Check sheet for the modelled part. Datum: model origin and axes. Units: mm. Face numbers are marked on the shaded views. A direction names the side the tool comes from. Give positions to 0.01 mm unless a question says otherwise; leave off trailing zeros. Loops run counter-clockwise (first coordinate to the right, second up) from the corner with the lowest first, then second, coordinate; pieces in that order, holes last. Notation, with made-up numbers: (-33, 6.25) - (15, 6.25) arc R16 ccw to (15, 17.25) - close; hole circle Ø1 at (39.25, 19). An arc over 180 degrees is marked (long way). Answer in a Markdown table with one row per item. Add a question column.
(1) Sectioned sample at D-D on x = -8.5. Enter the section's corners in (y, z) (3 decimals), then the cut area to 3 significant figures.
(2) Sectioned sample at A-A on z = 0. Enter the section's corners in (x, y) (3 decimals).
(3) Set-up check for the marked faces 5, 6 and 7: record each of +Z, -Z, +X, -X, +Y, -Y from which the full face is reachable in a straight line by a thin tool's end or side.
(4) Draft check along Z on the marked faces 1, 2, 3 and 4. Enter one of: released by +Z, released by -Z, zero draft, split by the parting line, or undercut.
(5) Thickness scan on L1, parallel to Z at x = 1, y = -37; L2, parallel to Y at x = 1.5, z = 20 (3 decimals); L3, parallel to Y at x = -7.75, z = -22.5 (3 decimals). Record the ranges inside material, lowest first.
(6) Sectioned sample at C-C on z = -23. Enter the section's corners in (x, y) (3 decimals), then the cut area to 3 significant figures.
(7) Sectioned sample at B-B on y = 21.5. Enter the section's corners in (x, z).
(8) Go/stop test with flat-tipped pins: P1, Ø15, axis at y = -47.075, z = -25, coming from the +X side; P2, Ø25, axis at y = 14, z = -3.5, coming from the -X side; P3, Ø12, axis at x = -4, y = -1.5, coming from the +Z side; P4, Ø6, axis at x = -4, z = 16.5, coming from the -Y side. Record where each tip stops, or that it passes through.
from build123d import *

# Parameters (mm, degrees)
SKETCH1_W           = 50
SKETCH1_H           = 66.15
SKETCH1_R           = 11
SKETCH1_R_2         = 1.55
BOSS_EXTRUDE1_DEPTH = 4
SKETCH2_W           = 50
SKETCH2_H           = 4
BOSS_EXTRUDE2_DEPTH = 38
CHAMFER1_SIZE       = 10
CHAMFER1_SIZE2      = 4.663076582
BOSS_EXTRUDE3_START = -18
SKETCH3_R           = 5.25
SKETCH3_R_2         = 1.4
BOSS_EXTRUDE3_DEPTH = 24
SKETCH4_W           = 18
SKETCH4_H           = 50
CUT_EXTRUDE1_DEPTH  = 24
FILLET1_R           = 10
SKETCH5_W           = 25
SKETCH5_H           = 15
CUT_EXTRUDE2_DEPTH  = 86.707383725


with BuildPart() as part:
    # Sketch1 → Boss-Extrude1 (new body)
    with BuildSketch(Plane(origin=(0, 0, 0), x_dir=(0, 0, -1), z_dir=(1, 0, 0))):
        Rectangle(SKETCH1_W, SKETCH1_H)
        with Locations((0, 11.925)):
            Circle(SKETCH1_R, mode=Mode.SUBTRACT)
        with Locations((-15.5, 27.425)):
            Circle(SKETCH1_R_2, mode=Mode.SUBTRACT)
        with Locations((15.5, 27.425)):
            Circle(SKETCH1_R_2, mode=Mode.SUBTRACT)
        with Locations((15.5, -3.575)):
            Circle(SKETCH1_R_2, mode=Mode.SUBTRACT)
        with Locations((-15.5, -3.575)):
            Circle(SKETCH1_R_2, mode=Mode.SUBTRACT)
    extrude(amount=BOSS_EXTRUDE1_DEPTH)

    # Sketch2 → Boss-Extrude2 (add)
    with BuildSketch(Plane.ZY):
        with Locations((0, -31.075)):
            Rectangle(SKETCH2_W, SKETCH2_H)
    extrude(amount=BOSS_EXTRUDE2_DEPTH)

    # Chamfer1
    chamfer1_edges = [part.edges().sort_by_distance(p)[0] for p in [
        (0, -29.075, 0),
    ]]
    chamfer1_side = [part.faces().sort_by_distance(p)[0] for p in [
        (0, 0.490102601, 0),
    ]]
    chamfer(chamfer1_edges, length=CHAMFER1_SIZE, length2=CHAMFER1_SIZE2, reference=chamfer1_side[0])

    # Sketch3 → Boss-Extrude3 (add)
    with BuildSketch(Plane.ZY.offset(38).offset(BOSS_EXTRUDE3_START)):
        with BuildLine():
            Line((-25, -33.075), (-25, -38.075))
            ThreePointArc((-25, -38.075), (-32.372368399, -41.912812073), (-33.457233587, -50.15318129))
            Line((-33.457233587, -50.15318129), (-31.108002035, -49.298130932))
            ThreePointArc((-31.108002035, -49.298130932), (-18.994783039, -44.58755769), (-30.891000616, -49.822018701))
            Line((-30.891000616, -49.822018701), (-33.156770083, -50.878564356))
            ThreePointArc((-33.156770083, -50.878564356), (-29.835696475, -54.665523012), (-25, -56.075))
            Line((-25, -56.075), (-7.705679723, -56.075))
            ThreePointArc((-7.705679723, -56.075), (0, -74.925), (7.705679723, -56.075))
            Line((7.705679723, -56.075), (25, -56.075))
            ThreePointArc((25, -56.075), (29.835696475, -54.665523012), (33.156770083, -50.878564356))
            Line((33.156770083, -50.878564356), (30.891000616, -49.822018701))
            ThreePointArc((30.891000616, -49.822018701), (18.994783039, -44.58755769), (31.108002035, -49.298130932))
            Line((31.108002035, -49.298130932), (33.457233587, -50.15318129))
            ThreePointArc((33.457233587, -50.15318129), (32.372368399, -41.912812073), (25, -38.075))
            Line((25, -38.075), (25, -33.075))
            Line((25, -33.075), (-25, -33.075))
        make_face()
        with Locations((0, -63.925)):
            Circle(SKETCH3_R, mode=Mode.SUBTRACT)
        with Locations((0, -55.925)):
            Circle(SKETCH3_R_2, mode=Mode.SUBTRACT)
        with Locations((-8, -63.925)):
            Circle(SKETCH3_R_2, mode=Mode.SUBTRACT)
        with Locations((0, -71.925)):
            Circle(SKETCH3_R_2, mode=Mode.SUBTRACT)
        with Locations((8, -63.925)):
            Circle(SKETCH3_R_2, mode=Mode.SUBTRACT)
    extrude(amount=-BOSS_EXTRUDE3_DEPTH)

    # Sketch4 → Cut-Extrude1 (cut)
    with BuildSketch(Plane.XZ.offset(33.075)):
        with Locations((-29, 0)):
            Rectangle(SKETCH4_W, SKETCH4_H)
    extrude(amount=-CUT_EXTRUDE1_DEPTH, mode=Mode.SUBTRACT)

    # Fillet1
    fillet1_edges = [part.edges().sort_by_distance(p)[0] for p in [
        (-8, -56.075, -7.705679723),
        (-8, -56.075, 7.705679723),
    ]]
    fillet(fillet1_edges, radius=FILLET1_R)

    # Sketch5 → Cut-Extrude2 (cut, through all)
    with BuildSketch(Plane.ZY.offset(20)):
        with Locations((0, -41.575)):
            Rectangle(SKETCH5_W, SKETCH5_H)
    extrude(amount=-CUT_EXTRUDE2_DEPTH, mode=Mode.SUBTRACT)


solid = part.part
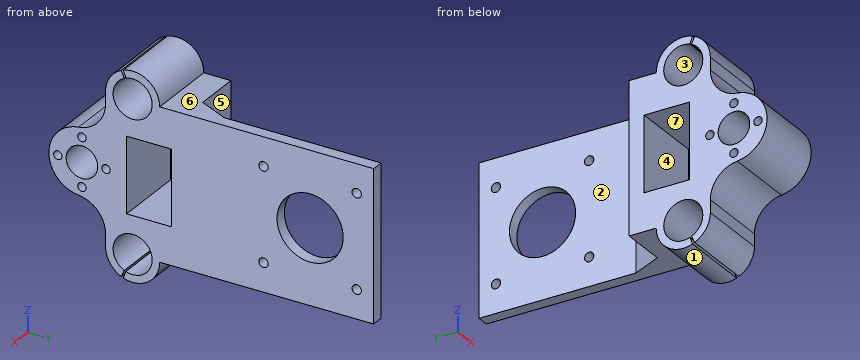
Reply:
| question | item | result |
|---|---|---|
| 1 | outline | (-65.051, -10.942) arc R10 cw to (-56.075, -20.89) - (-56.075, -25) arc R9 ccw to (-50.879, -33.157) - (-49.822, -30.891) arc R6.5 cw (long way) to (-49.298, -31.108) - (-50.153, -33.457) arc R9 ccw to (-38.075, -25) - (-29.075, -25) - (-29.075, 25) - (-38.075, 25) arc R9 ccw to (-50.153, 33.457) - (-49.298, 31.108) arc R6.5 cw (long way) to (-49.822, 30.891) - (-50.879, 33.157) arc R9 ccw to (-56.075, 25) - (-56.075, 20.89) arc R10 cw to (-65.051, 10.942) arc R11 ccw to start; hole circle Ø2.8 at (-71.925, 0); hole circle Ø10.5 at (-63.925, 0); hole circle Ø2.8 at (-63.925, -8); hole circle Ø2.8 at (-63.925, 8); hole circle Ø2.8 at (-55.925, 0); hole (-49.075, -12.5) - (-34.075, -12.5) - (-34.075, 12.5) - (-49.075, 12.5) - close |
| 1 | area | 1,250 mm^2 |
| 2 | outline | (-20, -74.925) - (4, -74.925) - (4, -73.325) - (-20, -73.325) - close; (-20, -70.525) - (4, -70.525) - (4, -69.175) - (-20, -69.175) - close; (-20, -58.675) - (4, -58.675) - (4, -57.325) - (-20, -57.325) - close; (-20, -54.525) - (4, -54.525) - (4, -49.075) - (-20, -49.075) - close; (-20, -34.075) - (4, -34.075) - (4, 0.925) - (0, 0.925) - (0, -19.075) - (-4.663, -29.075) - (-20, -29.075) - close; (0, 22.925) - (4, 22.925) - (4, 33.075) - (0, 33.075) - close |
| 3 | face 5 | +Z, -Z, -X, +Y |
| 3 | face 6 | +Z, +X, -X, +Y |
| 3 | face 7 | +X, -X |
| 4 | face 1 | released by -Z |
| 4 | face 2 | zero draft |
| 4 | face 3 | undercut |
| 4 | face 4 | undercut |
| 5 | L1 | -25 to -12.5, 12.5 to 25 |
| 5 | L2 | -56.115 to -51.228, -42.922 to 33.075 |
| 5 | L3 | -56.075 to -53.075, -41.075 to -29.075 |
| 6 | outline | (-20, -56.075) - (4, -56.075) - (4, -53.26) - (-20, -53.26) - close; (-20, -40.89) - (4, -40.89) - (4, 33.075) - (0, 33.075) - (0, -19.075) - (-4.663, -29.075) - (-20, -29.075) - close |
| 6 | area | 623 mm^2 |
| 7 | outline | (0, -25) - (4, -25) - (4, -5.41) - (0, -5.41) - close; (0, 5.41) - (4, 5.41) - (4, 25) - (0, 25) - close |
| 8 | P1 | x = 4 |
| 8 | P2 | x = 0 |
| 8 | P3 | z = 25 |
| 8 | P4 | y = -59.34 |
